Part model, mm, in its own coordinate system. Round coordinates to 2 decimals unless told otherwise and drop trailing zeros. Write each loop counter-clockwise with the first axis right and the second up, starting at its lowest first coordinate (ties: lowest second). Pieces come first, ordered by that corner, then holes. Notation, with made-up numbers: (-36.5, -20) -> (-23.5, -20) arc R28 cw to (-23.5, 8) -> close; hole circle Ø4 at (69.5, 71). An arc over 180 degrees is marked (long way). Return JSON: item names as keys, results as strings. Group by question number.
```python
from build123d import *

# Parameters (mm, degrees)
BOSS_EXTRUDE1_DEPTH = 300
SKETCH2_R           = 3
CUT_EXTRUDE1_DEPTH  = 4.5
SKETCH3_R           = 1.75
CUT_EXTRUDE2_DEPTH  = 301.166620396


with BuildPart() as part:
    # Sketch1 → Boss-Extrude1 (new body)
    with BuildSketch(Plane.XY):
        with BuildLine():
            Line((-5.6, 4), (5.6, 4))
            ThreePointArc((5.6, 4), (5.882842712, 3.882842712), (6, 3.6))
            Line((6, 3.6), (6, 2.8))
            Line((6, 2.8), (5.2, 2))
            Line((5.2, 2), (4.4, 2))
            Line((4.4, 2), (4.4, 1))
            Line((4.4, 1), (5.2, 1))
            Line((5.2, 1), (6, 0.2))
            Line((6, 0.2), (6, -3.6))
            ThreePointArc((6, -3.6), (5.882842712, -3.882842712), (5.6, -4))
            Line((5.6, -4), (-5.6, -4))
            ThreePointArc((-5.6, -4), (-5.882842712, -3.882842712), (-6, -3.6))
            Line((-6, -3.6), (-6, 0.2))
            Line((-6, 0.2), (-5.2, 1))
            Line((-5.2, 1), (-4.4, 1))
            Line((-4.4, 1), (-4.4, 2))
            Line((-4.4, 2), (-5.2, 2))
            Line((-5.2, 2), (-6, 2.8))
            Line((-6, 2.8), (-6, 3.6))
            ThreePointArc((-6, 3.6), (-5.882842712, 3.882842712), (-5.6, 4))
        make_face()
    extrude(amount=BOSS_EXTRUDE1_DEPTH)

    # Sketch2 → Cut-Extrude1 (cut)
    with BuildSketch(Plane(origin=(0, 4, 0), x_dir=(1, 0, 0), z_dir=(0, 1, 0))):
        with Locations(Location((0, -290, 0), (0, 0, 270))):
            Circle(SKETCH2_R)
        with Locations(Location((0, -265, 0), (0, 0, 270))):
            Circle(SKETCH2_R)
        with Locations(Location((0, -240, 0), (0, 0, 270))):
            Circle(SKETCH2_R)
        with Locations(Location((0, -215, 0), (0, 0, 270))):
            Circle(SKETCH2_R)
        with Locations(Location((0, -190, 0), (0, 0, 270))):
            Circle(SKETCH2_R)
        with Locations(Location((0, -165, 0), (0, 0, 270))):
            Circle(SKETCH2_R)
        with Locations(Location((0, -140, 0), (0, 0, 270))):
            Circle(SKETCH2_R)
        with Locations(Location((0, -115, 0), (0, 0, 270))):
            Circle(SKETCH2_R)
        with Locations(Location((0, -90, 0), (0, 0, 270))):
            Circle(SKETCH2_R)
        with Locations(Location((0, -65, 0), (0, 0, 270))):
            Circle(SKETCH2_R)
        with Locations(Location((0, -40, 0), (0, 0, 270))):
            Circle(SKETCH2_R)
        with Locations(Location((0, -15, 0), (0, 0, 270))):
            Circle(SKETCH2_R)
        with Locations((0, 10)):
            Circle(SKETCH2_R)
        with Locations((0, 35)):
            Circle(SKETCH2_R)
        with Locations((0, 60)):
            Circle(SKETCH2_R)
        with Locations((0, 85)):
            Circle(SKETCH2_R)
        with Locations((0, 110)):
            Circle(SKETCH2_R)
        with Locations((0, 135)):
            Circle(SKETCH2_R)
    extrude(amount=-CUT_EXTRUDE1_DEPTH, mode=Mode.SUBTRACT)

    # Sketch3 → Cut-Extrude2 (cut, through all)
    with BuildSketch(Plane(origin=(0, 4, 0), x_dir=(1, 0, 0), z_dir=(0, 1, 0))):
        with Locations(Location((0, -290.001504258, 0), (0, 0, 270))):
            Circle(SKETCH3_R)
        with Locations(Location((0, -265.001504258, 0), (0, 0, 270))):
            Circle(SKETCH3_R)
        with Locations(Location((0, -240.001504258, 0), (0, 0, 270))):
            Circle(SKETCH3_R)
        with Locations(Location((0, -215.001504258, 0), (0, 0, 270))):
            Circle(SKETCH3_R)
        with Locations(Location((0, -190.001504258, 0), (0, 0, 270))):
            Circle(SKETCH3_R)
        with Locations(Location((0, -165.001504258, 0), (0, 0, 270))):
            Circle(SKETCH3_R)
        with Locations(Location((0, -140.001504258, 0), (0, 0, 270))):
            Circle(SKETCH3_R)
        with Locations(Location((0, -115.001504258, 0), (0, 0, 270))):
            Circle(SKETCH3_R)
        with Locations(Location((0, -90.001504258, 0), (0, 0, 270))):
            Circle(SKETCH3_R)
        with Locations(Location((0, -65.001504258, 0), (0, 0, 270))):
            Circle(SKETCH3_R)
        with Locations(Location((0, -40.001504258, 0), (0, 0, 270))):
            Circle(SKETCH3_R)
        with Locations(Location((0, -15.001504258, 0), (0, 0, 270))):
            Circle(SKETCH3_R)
        with Locations((0, 9.998495742)):
            Circle(SKETCH3_R)
        with Locations((0, 34.998495742)):
            Circle(SKETCH3_R)
        with Locations((0, 59.998495742)):
            Circle(SKETCH3_R)
    extrude(amount=-CUT_EXTRUDE2_DEPTH, mode=Mode.SUBTRACT)


solid = part.part
```
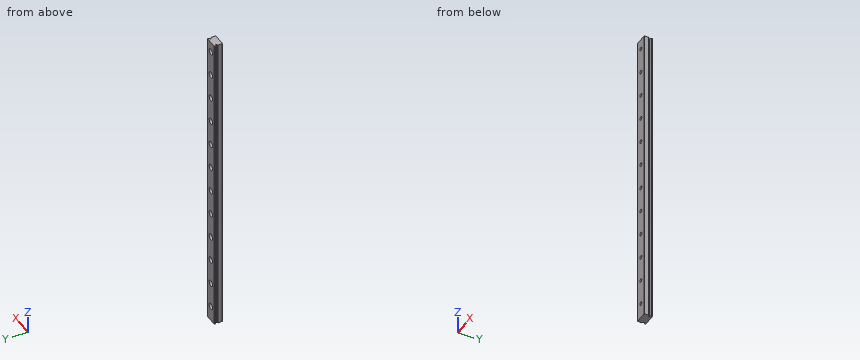
Item 1: Cut at B-B (z = 150). Write the cut outline in (x, y), then the cut area to 3 significant figures.
Item 2: Cut at A-A (y = -1.75). State how many separate pieces and enclosed holes the cut face has, then the cut area to 3 significant figures.
Item 3: Flat gauge pins, fed straight in: P1, Ø4.5, axis at x = 0, z = 115, coming from the -Y side; P2, Ø4, axis at x = 0, z = 140, coming from the +Y side; P3, Ø1.1, axis at y = 1.5, z = 187, coming from the +X side; P4, Ø2, axis at y = 1.5, z = 95, coming from the -X side. Where does each tip first touch, or does it go through?
Item 4: Wall check: L1, parallel to Y at x = -4.5, z = 139.5; L2, parallel to X at y = 2.95, z = 265; L3, parallel to Y at x = 5.25, z = 225. Give the ranges that are in metal, low to high.
Checks:
{
 "1": {"outline": "(-6, -3.6) arc R0.4 ccw to (-5.6, -4) -> (5.6, -4) arc R0.4 ccw to (6, -3.6) -> (6, 0.2) -> (5.2, 1) -> (4.4, 1) -> (4.4, 2) -> (5.2, 2) -> (6, 2.8) -> (6, 3.6) arc R0.4 ccw to (5.6, 4) -> (-5.6, 4) arc R0.4 ccw to (-6, 3.6) -> (-6, 2.8) -> (-5.2, 2) -> (-4.4, 2) -> (-4.4, 1) -> (-5.2, 1) -> (-6, 0.2) -> close", "area": "91.4 mm2"},
 "2": {"separate pieces": "1", "enclosed holes": "12", "area": "3,480 mm2"},
 "3": {"P1": "stops at y = -4", "P2": "stops at y = -0.5", "P3": "stops at x = 5.25", "P4": "stops at x = -5.7"},
 "4": {"L1": "y = -4 to 1, 2 to 4", "L2": "x = -6 to -3, 3 to 6", "L3": "y = -4 to 0.95, 2.05 to 4"}
}
